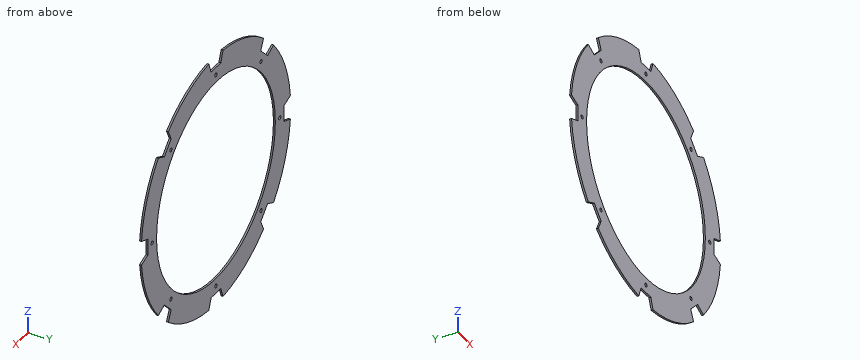
from build123d import *

# Parameters (mm, degrees)
SKETCH2_R             = 3.175
SKETCH2_R_2           = 171.45
BOSS_EXTRUDE1_DEPTH   = 3.175
CIRPATTERN1_OUTLINE_R = 3.175
CIRPATTERN1_DEPTH     = 3.175


# Read off the part's stored shape, not the designer's step: CirPattern1
with BuildPart() as part:
    # Sketch2 → Boss-Extrude1 (new body)
    with BuildSketch(Plane(origin=(0, 0, 0), x_dir=(1, 0, 0), z_dir=(0, 1, 0))):
        with BuildLine():
            Line((-214.920060182, 20.546964038), (-196.85, 13.97))
            Line((-196.85, 13.97), (-196.85, -13.97))
            Line((-196.85, -13.97), (-214.920060182, -20.546964038))
            ThreePointArc((-214.920060182, -20.546964038), (10.285159372, -215.654875894), (215.9, 0))
            ThreePointArc((215.9, 0), (10.285159372, 215.654875894), (-214.920060182, 20.546964038))
        make_face()
        with Locations(Location((-184.15, 0, 0), (0, 0, 270))):
            Circle(SKETCH2_R, mode=Mode.SUBTRACT)
        with Locations(Location((0, 0, 0), (0, 0, 270))):
            Circle(SKETCH2_R_2, mode=Mode.SUBTRACT)
    extrude(amount=BOSS_EXTRUDE1_DEPTH)

    # CirPattern1 outline → CirPattern1 (cut)
    with BuildSketch(Plane(origin=(0, 0, 0), x_dir=(1, 0, 0), z_dir=(0, 1, 0))):
        with BuildLine():
            Line((-129.315688143, 149.07225161), (-137.442534364, 166.500329572))
            ThreePointArc((-137.442534364, 166.500329572), (-152.664354058, 152.664354058), (-166.500329572, 137.442534364))
            Line((-166.500329572, 137.442534364), (-149.07225161, 129.315688143))
            Line((-149.07225161, 129.315688143), (-129.315688143, 149.07225161))
        make_face()
        with BuildLine():
            ThreePointArc((-166.500329572, -137.442534364), (-152.664354058, -152.664354058), (-137.442534364, -166.500329572))
            Line((-137.442534364, -166.500329572), (-129.315688143, -149.07225161))
            Line((-129.315688143, -149.07225161), (-149.07225161, -129.315688143))
            Line((-149.07225161, -129.315688143), (-166.500329572, -137.442534364))
        make_face()
        with BuildLine():
            ThreePointArc((-20.546964038, -214.920060182), (0, -215.9), (20.546964038, -214.920060182))
            Line((20.546964038, -214.920060182), (13.97, -196.85))
            Line((13.97, -196.85), (-13.97, -196.85))
            Line((-13.97, -196.85), (-20.546964038, -214.920060182))
        make_face()
        with BuildLine():
            ThreePointArc((137.442534364, -166.500329572), (152.664354058, -152.664354058), (166.500329572, -137.442534364))
            Line((166.500329572, -137.442534364), (149.07225161, -129.315688143))
            Line((149.07225161, -129.315688143), (129.315688143, -149.07225161))
            Line((129.315688143, -149.07225161), (137.442534364, -166.500329572))
        make_face()
        with BuildLine():
            ThreePointArc((214.920060182, -20.546964038), (215.9, 0), (214.920060182, 20.546964038))
            Line((214.920060182, 20.546964038), (196.85, 13.97))
            Line((196.85, 13.97), (196.85, -13.97))
            Line((196.85, -13.97), (214.920060182, -20.546964038))
        make_face()
        with BuildLine():
            ThreePointArc((166.500329572, 137.442534364), (152.664354058, 152.664354058), (137.442534364, 166.500329572))
            Line((137.442534364, 166.500329572), (129.315688143, 149.07225161))
            Line((129.315688143, 149.07225161), (149.07225161, 129.315688143))
            Line((149.07225161, 129.315688143), (166.500329572, 137.442534364))
        make_face()
        with BuildLine():
            ThreePointArc((20.546964038, 214.920060182), (0, 215.9), (-20.546964038, 214.920060182))
            Line((-20.546964038, 214.920060182), (-13.97, 196.85))
            Line((-13.97, 196.85), (13.97, 196.85))
            Line((13.97, 196.85), (20.546964038, 214.920060182))
        make_face()
        with Locations((-130.213713756, 130.213713756)):
            Circle(CIRPATTERN1_OUTLINE_R)
        with Locations((0, 184.15)):
            Circle(CIRPATTERN1_OUTLINE_R)
        with Locations((130.213713756, 130.213713756)):
            Circle(CIRPATTERN1_OUTLINE_R)
        with Locations((184.15, 0)):
            Circle(CIRPATTERN1_OUTLINE_R)
        with Locations((130.213713756, -130.213713756)):
            Circle(CIRPATTERN1_OUTLINE_R)
        with Locations((0, -184.15)):
            Circle(CIRPATTERN1_OUTLINE_R)
        with Locations((-130.213713756, -130.213713756)):
            Circle(CIRPATTERN1_OUTLINE_R)
    extrude(amount=CIRPATTERN1_DEPTH, mode=Mode.SUBTRACT)


solid = part.part
Verification items for the finished model (mm, model axes). Give positions to 0.01 mm unless a question says otherwise; leave off trailing zeros. Write each loop counter-clockwise with the first axis right and the second up, starting at its lowest first coordinate (ties: lowest second). Pieces come first, ordered by that corner, then holes.
(1) Cross-section at A-A (x = 89). Enter the section's corners in (y, z) (3 decimals).
(2) Gauge pin test, flat ends, axial feed: pin 1 (4 mm diameter, centred on x = -184.15, z = 0, fed in from -Y); pin 2 (1.6 mm diameter, centred on y = 1.5, z = -3, fed in from -X). Record the tip position at first contact, or that the pin passes through.
(3) Cross-section at B-B (z = -64). Enter the section's corners in (x, y) (3 decimals).
(4) Material ranges on line 1 (X direction, y = 1.3, z = 0) (3 decimals); line 2 (X direction, y = 1.2, z = 5); line 3 (X direction, y = 1.25, z = -114), recorded low to high.
(5) Cross-section at C-C (y = 0.7). State how many separate pieces and enclosed holes the cut face has, plus the area to 3 significant figures.
Worked out:
1. outline: (0, -196.702) - (3.175, -196.702) - (3.175, -146.54) - (0, -146.54) - close; (0, 146.54) - (3.175, 146.54) - (3.175, 196.702) - (0, 196.702) - close
2. pin 1: passes through
2. pin 2: stops at x = -196.85
3. outline: (-206.196, 0) - (-159.057, 0) - (-159.057, 3.175) - (-206.196, 3.175) - close; (159.057, 0) - (206.196, 0) - (206.196, 3.175) - (159.057, 3.175) - close
4. line 1: x = -196.85 to -187.325, -180.975 to -171.45, 171.45 to 180.975, 187.325 to 196.85
4. line 2: x = -196.85 to -171.38, 171.38 to 196.85
4. line 3: x = -183.35 to -128.06, 128.06 to 183.35
5. separate pieces: 1
5. enclosed holes: 9
5. area: 48,600 mm2
